```python
from build123d import *

# Parameters (mm, degrees)
F0_W      = 76.2
F0_H      = 76.2
F1_DEPTH  = 25.4
F2_R      = 2.54
F3_R      = 31.75
F3_R_2    = 29.21
F4_DEPTH  = 1.27
F5_D      = 5.08
F4_FACE_R = 29.21
F6_DEPTH  = 1.27
F7_R      = 24.13
F8_DEPTH  = 24.13
F9_D      = 43.18
F11_D     = 1.27
F11_DEPTH = 25.4


with BuildPart() as f1:
    # F0 (on Top) → F1 (new body)
    with BuildSketch(Plane.XY):
        Rectangle(F0_W, F0_H)
    extrude(amount=F1_DEPTH)

    # F2
    f2_edges = [f1.edges().sort_by_distance(p)[0] for p in [
        (38.1, -38.1, 12.7),
        (38.1, 38.1, 12.7),
        (-38.1, -38.1, 12.7),
        (-38.1, 38.1, 12.7),
    ]]
    fillet(f2_edges, radius=F2_R)

    # F3 (on face) → F4 (cut)
    with BuildSketch(Plane.XY.offset(25.4)):
        Circle(F3_R)
        Circle(F3_R_2, mode=Mode.SUBTRACT)
    extrude(amount=-F4_DEPTH, mode=Mode.SUBTRACT)

    # F5 (through all)
    with Locations(Plane.XY.offset(25.4)):
        with Locations((-31.75, 31.75), (31.75, 31.75), (31.75, -31.75), (-31.75, -31.75)):
            Hole(F5_D / 2)

    # F4_face (on face) → F6 (join)
    with BuildSketch(Plane.XY.offset(25.4)):
        Circle(F4_FACE_R)
    extrude(amount=F6_DEPTH)

    # F7 (on face) → F8 (cut)
    with BuildSketch(Plane(origin=(0, 0, 0), x_dir=(1, 0, 0), z_dir=(0, 0, -1))):
        Circle(F7_R)
    extrude(amount=-F8_DEPTH, mode=Mode.SUBTRACT)

    # F9 (through all)
    with Locations(Plane(origin=(0, 0, 0), x_dir=(1, 0, 0), z_dir=(0, 0, -1))):
        with Locations((0, 0)):
            Hole(F9_D / 2)

    # F11
    with Locations(Plane.XZ.offset(38.1)):
        with Locations((0, 19.05)):
            Hole(F11_D / 2, depth=F11_DEPTH)


solid = f1.part
```
Here's how the part is built. I have some questions about the finished solid (model axes, mm). A direction names the side the tool comes from. Coordinates: 2 decimals unless noted, no trailing zeros. Loops run counter-clockwise (first coordinate to the right, second up) from the corner with the lowest first, then second, coordinate; pieces in that order, holes last. Notation, with made-up numbers: (-23.5, 65) - (-2.5, 65) arc R26 cw to (-2.5, 91) - close; hole circle Ø2 at (81.5, 62). An arc over 180 degrees is marked (long way). Return JSON: item names as keys, results as strings. Group by question number.
Item 1: If we section it at A-A on y = 0: Write out the boundary of the cut face in (x, z).
Item 2: We'd pull the mould along Y, two halves only. Please class faces 4 (the face through (37.336, -37.376, 12.878)), 5 (the face through (-38.1, 0, 13)), 6 (the face through (23.016, -7.248, 11.896)): +Y half, -Y half, draft (parallel to the pull), parting line (faces both ways), or undercut.
Item 3: I need wall thicknesses on line 1 (Y direction, x = 31.5, z = 19); line 2 (Y direction, x = -33, z = 12.25); line 3 (Z direction, x = 0, y = -28.5) (3 decimals). Which ranges of each line are inside material? Lowest first, please. Write a range as from..to.
Item 4: On a 3-axis mill with a long thin cutter (end or side, diameter ignored), from which of +Z, -Z, +X, -X, +Y, -Y can I reach the whole of each face in a straight line? I mean faces 1 (the face through (-6.883, -30.995, 24.774)), 2 (the face through (-18, 12.4, 24.13)), 3 (the face through (0, -38.1, 13)). Say none if no direction works.
Item 5: If we section it at B-B on z = 8: Write out the boundary of the cut face in (x, y).
Item 6: Will these pins go through, and if not, where does the flat tip stop? P1, Ø4.5, axis at x = 31.75, y = -31.75, coming from the +Z side; P2, Ø0.8, axis at x = 0, z = 19.05, coming from the -Y side.
Item 7: If we section it at C-C on x = 9: Write out the boundary of the cut face in (y, z).
Calculated:
{
 "1": {"outline": "(-38.1, 0) - (-24.13, 0) - (-24.13, 24.13) - (-21.59, 24.13) - (-21.59, 26.67) - (-29.21, 26.67) - (-29.21, 24.13) - (-31.75, 24.13) - (-31.75, 25.4) - (-38.1, 25.4) - close; (21.59, 24.13) - (24.13, 24.13) - (24.13, 0) - (38.1, 0) - (38.1, 25.4) - (31.75, 25.4) - (31.75, 24.13) - (29.21, 24.13) - (29.21, 26.67) - (21.59, 26.67) - close"},
 "2": {"face 4": "-Y half", "face 5": "draft", "face 6": "undercut"},
 "3": {"line 1": "y = -38.1..-34.28, -29.22..29.22, 34.28..38.1", "line 2": "y = -38.1..-33.96, -29.54..29.54, 33.96..38.1", "line 3": "z = 0..18.415, 19.685..26.67"},
 "4": {"face 1": "+Z", "face 2": "-Z", "face 3": "+Z, -Z, +X, -X, -Y"},
 "5": {"outline": "(-38.1, -35.56) arc R2.54 ccw to (-35.56, -38.1) - (35.56, -38.1) arc R2.54 ccw to (38.1, -35.56) - (38.1, 35.56) arc R2.54 ccw to (35.56, 38.1) - (-35.56, 38.1) arc R2.54 ccw to (-38.1, 35.56) - close; hole circle Ø5.08 at (-31.75, -31.75); hole circle Ø5.08 at (-31.75, 31.75); hole circle Ø48.26 at (0, 0); hole circle Ø5.08 at (31.75, -31.75); hole circle Ø5.08 at (31.75, 31.75)"},
 "6": {"P1": "passes through", "P2": "stops at y = 24.13"},
 "7": {"outline": "(-38.1, 0) - (-22.39, 0) - (-22.39, 24.13) - (-19.62, 24.13) - (-19.62, 26.67) - (-27.79, 26.67) - (-27.79, 24.13) - (-30.45, 24.13) - (-30.45, 25.4) - (-38.1, 25.4) - close; (19.62, 24.13) - (22.39, 24.13) - (22.39, 0) - (38.1, 0) - (38.1, 25.4) - (30.45, 25.4) - (30.45, 24.13) - (27.79, 24.13) - (27.79, 26.67) - (19.62, 26.67) - close"}
}
